Autodesk Inventor part; units mm, degrees
ref_plane "YZ Plane" through (0, 0, 0) normal (1, 0, 0) x (0, 1, 0)
ref_plane "XZ Plane" through (0, 0, 0) normal (0, 1, 0) x (-1, 0, 0)
ref_plane "XY Plane" through (0, 0, 0) normal (0, 0, 1) x (1, 0, 0)
sketch "Sketch1" plane through (0, 0, 0) normal (0, 0, 1) x (1, 0, 0)
  circle A0 centre (0, 0) radius 30.226
  line L0 (30.226, 0) -> (55.626, 0)
  line L1 (55.626, 0) -> (55.626, 63.5)
  line L2 (55.626, 63.5) -> (-103.124, 63.5)
  line L3 (-28.4673, 10.16) -> (-103.124, 10.16)
  line L4 (-103.124, 10.16) -> (-103.124, 63.5)
  arc A1 (-103.124, 63.5) -> (-28.4673, 10.16) centre (-32.2937, 83.7205) ccw
  point P0 (-36.1202, 10.16)
  dimension "d0" = 60.452
  dimension "d1" = 25.4
  dimension "d2" = 63.5
  dimension "d3" = 158.75
  dimension "d4" = 53.34
  dimension "d7" = 73.66
extrude "Extrusion1" add sketch "Sketch1" along normal blind 1.5875 contours A0 L3 A1 L2 L1 L0
sketch "Sketch2" plane through (0, 0, 1.5875) normal (0, 0, 1) x (1, 0, 0)
  line L0 (50.5354, 58.4509) -> (55.6154, 58.4509)
  line L1 (50.5354, 58.4509) -> (50.5354, 63.5309)
  circle A0 centre (50.5354, 58.4509) radius 2.54
  line L2 (50.5354, 58.4509) -> (50.5354, 33.0509)
  circle A1 centre (50.5354, 33.0509) radius 2.54
  line L3 (50.5354, 33.0509) -> (50.5354, 7.6509)
  circle A2 centre (50.5354, 7.6509) radius 2.54
  line L4 (50.5354, 58.4509) -> (25.1354, 58.4509)
  circle A3 centre (25.1354, 58.4509) radius 2.54
  line L5 (25.1354, 58.4509) -> (-0.2646, 58.4509)
  circle A4 centre (-0.2646, 58.4509) radius 2.54
  line L6 (-0.2646, 58.4509) -> (-89.1646, 58.4509)
  circle A5 centre (-89.1646, 58.4509) radius 2.54
  line L7 (50.5354, 33.0509) -> (-76.4646, 33.0509)
  circle A6 centre (-76.4646, 33.0509) radius 2.54
  line L8 (50.5354, 20.3509) -> (-51.0646, 20.3509)
  circle A7 centre (-51.0646, 20.3509) radius 2.54
  point P0 (0, 0)
  dimension "d16" = 5.08
  dimension "d17" = 25.4
  dimension "d18" = 5.08
  dimension "d19" = 25.4
  dimension "d20" = 5.08
  dimension "d21" = 25.4
  dimension "d22" = 5.08
  dimension "d23" = 25.4
  dimension "d24" = 5.08
  dimension "d25" = 88.9
  dimension "d26" = 5.08
  dimension "d29" = 127
  dimension "d30" = 5.08
  dimension "d31" = 101.6
  dimension "d32" = 5.08
extrude "Extrusion2" cut sketch "Sketch2" against normal blind 25.4
fillet "Fillet1" radius 3.175 4 edges at (-103.124, 63.5, 0.7937) (55.626, 0, 0.7937) (30.226, 0, 0.7937) (55.626, 63.5, 0.7937)
fillet "Fillet2" radius 3.175 1 edges at (-28.4673, 10.16, 0.7937)
properties part number "Horizontal climb"
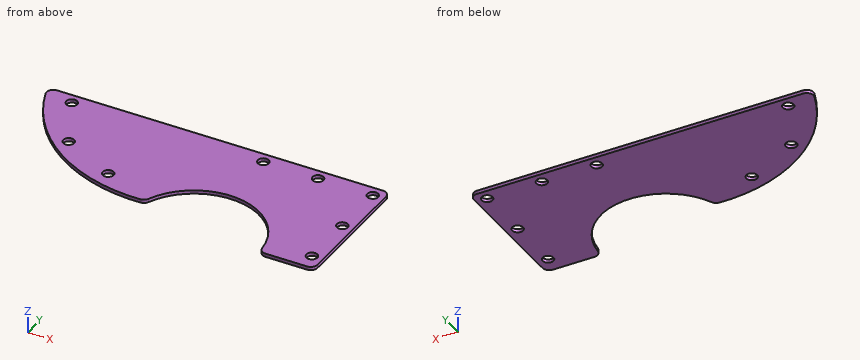
The listing builds one solid part. Answer for the finished solid, in the listing's coordinates (mm). Coordinates: 2 decimals unless noted, no trailing zeros. Write each loop counter-clockwise with the first axis right and the second up, starting at its lowest first coordinate (ties: lowest second). Pieces come first, ordered by that corner, then holes. Notation, with made-up numbers: (-22.75, 67) - (32.25, 67) arc R27 ccw to (32.25, 106) - close; hole circle Ø9 at (-20.5, -11). An arc over 180 degrees is marked (long way). One line per item, written item: value.
1) Find section A-A (y = 27). Give the vertices of the cut face in (x, z).
Geometry check:
outline: (-79.29, 0) - (-13.59, 0) - (-13.59, 1.59) - (-79.29, 1.59) - close; (13.59, 0) - (55.63, 0) - (55.63, 1.59) - (13.59, 1.59) - close
2) This flat-tipped pin is pushed along its axis until it touches: pin 1 Ø8 at (x, y) = (-0.26, 58.45) entering from -Z. Where does it stop, or does it pass through?
Geometry check:
pin 1: stops at z = 0
3) Find section B-B (z = 0.8). Count the separate pieces of the cut face and the enclosed holes in it, and give its area (3 significant figures).
Geometry check:
separate pieces: 1
enclosed holes: 8
area: 6,740 mm2
4) Consider line 1 along X through (y, z) = (22.5, 0.7); line 2 along X through (y, z) = (21, 0.55); line 3 along X through (y, z) = (17, 0.7). Determine where each line is inside the solid, lowest interval first. Write a range as from..to.
Geometry check:
line 1: x = -73.26..-52.42, -49.71..-20.18, 20.18..55.63
line 2: x = -70.92..-53.52, -48.61..-21.74, 21.74..55.63
line 3: x = -63.51..-24.99, 24.99..55.63
5) Find section D-D (y = 38.5). Give the vertices of the cut face in (x, z).
Geometry check:
outline: (-90.44, 0) - (55.63, 0) - (55.63, 1.59) - (-90.44, 1.59) - close
6) Find section C-C (x = -34). Give the vertices of the cut face in (y, z), and give its area (3 significant figures).
Geometry check:
outline: (10.16, 0) - (63.5, 0) - (63.5, 1.59) - (10.16, 1.59) - close
area: 84.7 mm2
